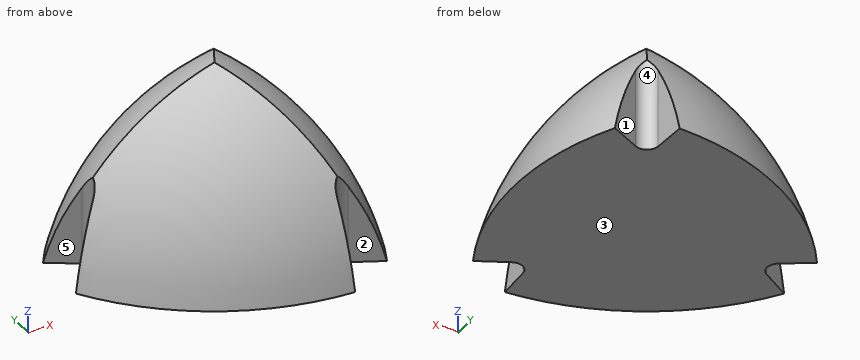
Autodesk Inventor part; units mm, degrees
ref_plane "YZ Plane" through (0, 0, 0) normal (1, 0, 0) x (0, 1, 0)
ref_plane "XZ Plane" through (0, 0, 0) normal (0, 1, 0) x (-1, 0, 0)
ref_plane "XY Plane" through (0, 0, 0) normal (0, 0, 1) x (1, 0, 0)
sketch "Sketch1" plane through (0, 0, 0) normal (0, 0, 1) x (1, 0, 0)
  circle A0 centre (0, 0) radius 500
  dimension "d0" = 1000
extrude "Extrusion1" add sketch "Sketch1" along normal blind 1000
sketch "Sketch2" plane through (0, 0, 0) normal (0, 1, 0) x (-1, 0, 0)
  line L0 (144.3376, 0) -> (-72.1688, -125)
  line L1 (-72.1688, -125) -> (-72.1688, 125)
  line L2 (-72.1688, 125) -> (144.3376, 0)
  line L3 (144.3376, 0) -> (144.3376, -72)
  arc A0 (144.3376, 223) -> (144.3376, -367) centre (144.3376, -72) ccw
  line L4 (144.3376, 0) -> (144.3376, 223)
  line L5 (144.3376, -72) -> (144.3376, -367)
  line L6 (144.3376, -367) -> (144.3376, 223)
  line L7 (144.3376, -367) -> (-768.1743, -367)
  line L8 (-768.1743, -367) -> (-768.1743, 1365.1918)
  line L9 (-768.1743, 1365.1918) -> (144.3376, 1365.1918)
  line L10 (144.3376, 1365.1918) -> (144.3376, 223)
  point P0 (0, 0)
  point P1 (0, 0)
  dimension "d4" = 250
  dimension "d5" = 72
  dimension "d6" = 590
  dimension "d7" = 1732.1918
  dimension "d8" = 912.5119
revolve "Revolution1" cut sketch "Sketch2" angle 360 about axis through (-144.3376, 0, 1365.1918) along (0, 0, -1) contours A0 L7 L8 L9 L10
pattern_circular "Circular Pattern1" count 3 over 360 about axis through (0, 0, -10) along (0, 0, 1) of "Revolution1"
sketch "Sketch3" plane through (0, 0, 0) normal (0, 0, -1) x (-1, 0, 0)
  arc A0 (-92.578, -160.3497) -> (185.1559, 0) centre (-72.1688, 125) ccw
  arc A1 (185.1559, 0) -> (-92.578, 160.3497) centre (-72.1688, -125) ccw
  arc A2 (-92.578, 160.3497) -> (-92.578, -160.3497) centre (144.3376, 0) ccw
  circle A3 centre (-72.1688, 125) radius 12.5
  line L0 (-110.2559, 130.4728) -> (-77.8697, 113.8757)
  line L1 (-59.6844, 124.375) -> (-57.8649, 160.7208)
  point P0 (0, 0)
  dimension "d13" = 25
extrude "Extrusion2" cut sketch "Sketch3" against normal blind 1000 contours A2 A1 L1 A3 L0 | A3
pattern_circular "Circular Pattern2" count 3 over 360 about axis through (0, 0, -10) along (0, 0, 1) of "Extrusion2"
properties part number "WORK ENVELOPE"
Read the model definition and answer for the solid it produces. Units are mm, in the model's axes. Face numbers are marked on the shaded views. A direction names the side the tool comes from. Round coordinates to 2 decimals unless told otherwise and drop trailing zeros. Write each loop counter-clockwise with the first axis right and the second up, starting at its lowest first coordinate (ties: lowest second). Pieces come first, ordered by that corner, then holes.
Q1. Find section A-A on z = 36.5. Determine the outline of the cut face in (x, y) (3 decimals).
Values:
outline: (-158.246, -23.868) arc R274.322 ccw to (58.453, -148.979) - (59.684, -124.375) arc R12.5 cw to (77.87, -113.876) - (99.793, -125.111) arc R274.322 ccw to (99.793, 125.111) - (77.87, 113.876) arc R12.5 cw to (59.684, 124.375) - (58.453, 148.979) arc R274.322 ccw to (-158.246, 23.868) - (-137.554, 10.499) arc R12.5 cw to (-137.554, -10.499) - close
Q2. Straight lines are drawn through the part: line 1 (X direction, y = -128, z = 10); line 2 (Y direction, x = 38, z = 107.5); line 3 (Z direction, x = -60.5, y = 76). For each, find the intervals that lie inside material, in ascending order.
Values:
line 1: x = -55.47 to 59.5, 105.43 to 108.48
line 2: y = -106.6 to 106.6
line 3: z = 0 to 98.36
Q3. Find section B-B on x = 89. Determine the outline of the cut face in (y, z), and give its area (3 significant figures).
Values:
outline: (-119.58, 0) - (119.58, 0) - (119.58, 63.2) arc R180.5 ccw to (-119.58, 63.2) - close
area: 22,500 mm2
Q4. Flat-ended cylindrical pins translate along their axes: P1, Ø1.5, axis at y = 118, z = 43.5, coming from the +X side; P2, Ø1, axis at y = 80, z = 81.5, coming from the +X side; P3, Ø1.5, axis at x = 8, z = 92.5, coming from the +Y side. Find the tip coordinate at first contact, or state that the pin passes through.
Values:
P1: stops at x = 100.63
P2: stops at x = 94.9
P3: stops at y = 111.88
Q5. Find section C-C on y = -18.5. Determine the outline of the cut face in (x, z), and give its area (3 significant figures).
Values:
outline: (-149.94, 0) - (141.14, 0) arc R294.42 ccw to (10.68, 178.3) arc R257.75 ccw to (-149.94, 58.77) - close
area: 36,600 mm2
Q6. Find section D-D on z = 91. Determine the outline of the cut face in (x, y).
Values:
outline: (-134.68, -7.93) arc R245.88 ccw to (60.47, -120.6) arc R12.5 cw to (74.21, -112.67) arc R245.88 ccw to (74.21, 112.67) arc R12.5 cw to (60.47, 120.6) arc R245.88 ccw to (-134.68, 7.93) arc R12.5 cw to start
Q7. A tool of negligible diameter and unlimited length cuts with its end or side. For the marked faces 1 and 2, from which of +Z, -Z, +X, -X, +Y, -Y can it reach the whole face along a straight path? Write none if from no direction.
Values:
face 1: +Z, -Z, +Y
face 2: +Z, -Z, -Y
Q8. The mould has two halves that part along X. Classify the marked faces 3, 4 and 5: released by +X, released by -X, zero draft, split by the parting line, or undercut.
Values:
face 3: zero draft
face 4: undercut
face 5: released by -X
